from build123d import *

# Parameters (mm, degrees)
SKETCH004_W      = 15
SKETCH004_H      = 435
EXTRUDE004_DEPTH = 780
ARRAY_X_COUNT    = 3
ARRAY_X_PITCH    = 1207.5
SKETCH003_W      = 2430
SKETCH003_H      = 435
EXTRUDE003_DEPTH = 15
ARRAY002_Z_COUNT = 3
ARRAY002_Z_PITCH = 260


with BuildPart() as obj1:
    # Sketch004 → Extrude004 (new body)
    with BuildSketch(Plane.XY):
        with Locations((7.5, 217.5)):
            Rectangle(SKETCH004_W, SKETCH004_H)
    extrude(amount=EXTRUDE004_DEPTH)

    # Array X: obj1 ×3


with BuildPart() as obj1_1:
    add(obj1.part)
    with Locations(*[(i * ARRAY_X_PITCH, 0, 0) for i in range(1, ARRAY_X_COUNT)]):
        add(obj1.part)


with BuildPart() as obj1_2:
    # Array placement: moved
    add(obj1_1.part.moved(Location((20, 15, 35))))


with BuildPart() as obj2:
    # Sketch003 → Extrude003 (new body)
    with BuildSketch(Plane.XY):
        with Locations((1215, 217.5)):
            Rectangle(SKETCH003_W, SKETCH003_H)
    extrude(amount=EXTRUDE003_DEPTH)


with BuildPart() as obj2_1:
    # Extrude003 placement: moved
    add(obj2.part.moved(Location((20, 15, 20))))

    # Array002 Z: obj2 ×3


with BuildPart() as obj2_2:
    add(obj2_1.part)
    with Locations(*[(0, 0, i * ARRAY002_Z_PITCH) for i in range(1, ARRAY002_Z_COUNT)]):
        add(obj2_1.part)

    # Fusion001: union obj1
    add(obj1_2.part)


solid = obj2_2.part
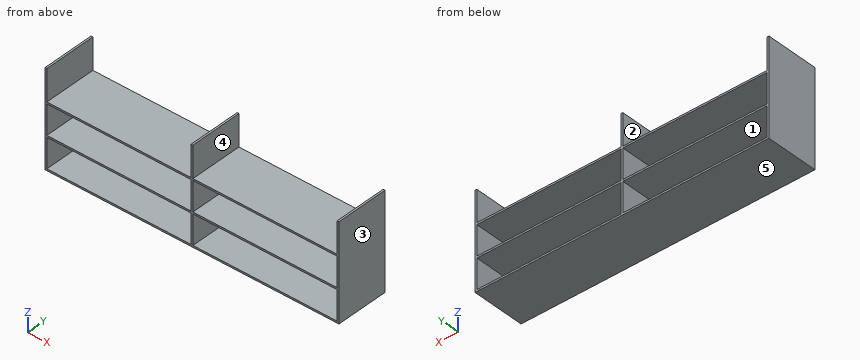
Source: CAD feature listing. Evaluate the final solid. Frame: model axes, mm. Face numbers are marked on the shaded views. A direction names the side the tool comes from. Round coordinates to 2 decimals unless told otherwise and drop trailing zeros. Order: outer loops, then holes, each group sorted by start corner. A loop starts at its lowest first (then second) coordinate and runs counter-clockwise, first axis right, second up. Notation, with made-up numbers: (13.5, -16.5) -> (63.5, -16.5) arc R16 ccw to (63.5, 8.5) -> close; hole circle Ø6 at (40, -34). An arc over 180 degrees is marked (long way). Answer as CSV lines item,"result".
Item 1: Reachability of the marked faces 1 and 2 from +Z, -Z, +X, -X, +Y, -Y: full face, straight path, thin tool, end or side. Return the list, or none.
A:
face 1,"+Y, -Y"
face 2,"+Z, +Y, -Y"
Item 2: Section B-B, the plane y = 223. Return loops of the section in (x, z).
A:
outline,"(20, 20) -> (2450, 20) -> (2450, 815) -> (2435, 815) -> (2435, 555) -> (1242.5, 555) -> (1242.5, 815) -> (1227.5, 815) -> (1227.5, 555) -> (35, 555) -> (35, 815) -> (20, 815) -> close; hole (35, 35) -> (1227.5, 35) -> (1227.5, 280) -> (35, 280) -> close; hole (35, 295) -> (1227.5, 295) -> (1227.5, 540) -> (35, 540) -> close; hole (1242.5, 35) -> (2435, 35) -> (2435, 280) -> (1242.5, 280) -> close; hole (1242.5, 295) -> (2435, 295) -> (2435, 540) -> (1242.5, 540) -> close"
Item 3: Line query: L1, parallel to Z at x = 1208.5, y = 393.5; L2, parallel to X at y = 374, z = 419. Output: solid intervals per line, ascending.
A:
L1,"20 to 35, 280 to 295, 540 to 555"
L2,"20 to 35, 1227.5 to 1242.5, 2435 to 2450"
Item 4: Pin query (flat end, axial travel): pin 1 Ø8 at (x, y) = (2048, 185.5) entering from +Z. Return the tip coordinate at first contact, or that it passes through.
A:
pin 1,"z = 555"
Item 5: Section C-C, the plane x = 275.5. Return loops of the section in (y, z), plus the area to 3 significant figures.
A:
outline,"(15, 20) -> (450, 20) -> (450, 35) -> (15, 35) -> close; (15, 280) -> (450, 280) -> (450, 295) -> (15, 295) -> close; (15, 540) -> (450, 540) -> (450, 555) -> (15, 555) -> close"
area,"19,600 mm²"
Item 6: Section A-A, the plane z = 606.5. Return loops of the section in (x, y), plus the area to 3 significant figures.
A:
outline,"(20, 15) -> (35, 15) -> (35, 450) -> (20, 450) -> close; (1227.5, 15) -> (1242.5, 15) -> (1242.5, 450) -> (1227.5, 450) -> close; (2435, 15) -> (2450, 15) -> (2450, 450) -> (2435, 450) -> close"
area,"19,600 mm²"
Item 7: Pull-direction query (X, two-part tool) for the marked faces 3, 4 and 5; classes: pulls with the +X half, pulls with the -X half, needs draft (parallel to the pull), parting line crosses it, or undercut.
A:
face 3,"pulls with the +X half"
face 4,"undercut"
face 5,"needs draft"
